Autodesk Inventor part; units mm, degrees
ref_plane "YZ Plane" through (0, 0, 0) normal (1, 0, 0) x (0, 1, 0)
ref_plane "XZ Plane" through (0, 0, 0) normal (0, 1, 0) x (-1, 0, 0)
ref_plane "XY Plane" through (0, 0, 0) normal (0, 0, 1) x (1, 0, 0)
sketch "Sketch1" plane through (0, 0, 0) normal (0, 0, 1) x (1, 0, 0)
  line L0 (-15, 70.8) -> (15, 70.8)
  line L1 (15, 70.8) -> (15, -70.8)
  line L2 (15, -70.8) -> (-15, -70.8)
  line L3 (-15, -70.8) -> (-15, 70.8)
  line L4 (0, 70.8) -> (0, -70.8) construction
  line L5 (-15, 58.8) -> (15, 58.8)
  line L6 (15, 58.8) -> (15, -58.8)
  line L7 (15, -58.8) -> (-15, -58.8)
  line L8 (-15, -58.8) -> (-15, 58.8)
  line L9 (0, 58.8) -> (0, -58.8) construction
  line L10 (-15, 58) -> (15, 58)
  line L11 (15, 58) -> (15, -58)
  line L12 (15, -58) -> (-15, -58)
  line L13 (-15, -58) -> (-15, 58)
  line L14 (0, 58) -> (0, -58) construction
  point P0 (0, 0)
  point P1 (0, 0)
  point P2 (15, -58)
  point P3 (-15, -58)
  point P4 (-15, -58.8)
  point P5 (15, -58.8)
  point P6 (-15, 58)
  point P7 (15, 58)
  point P8 (15, 58.8)
  point P9 (-15, 58.8)
  dimension "d0" = 141.6
  dimension "d1" = 30
  dimension "d4" = 117.6
  dimension "d5" = 116
extrude "Extrusion1" add sketch "Sketch1" against normal blind 0.6
extrude "Extrusion2" add sketch "Sketch1" along normal blind 5.2 contours L5 L1 L10 L3 | L12 L1 L7 L3
ref_plane "upper Plane" through (0, 0, 5.2) normal (0, 0, 1) x (1, 0, 0)
sketch "Sketch2" plane through (0, 0, 5.2) normal (0, 0, 1) x (1, 0, 0)
  line L0 (-15, 70.8) -> (15, 70.8)
  line L1 (-15, 70.8) -> (-15, 58.8)
  line L2 (-15, 58) -> (-15, -58)
  line L3 (-15, -58) -> (-15, -58.8)
  line L4 (-15, -58.8) -> (-15, -70.8)
  line L5 (-15, -70.8) -> (15, -70.8)
  line L6 (15, -70.8) -> (15, -58.8)
  line L7 (15, -58.8) -> (15, -58)
  line L8 (15, -58) -> (15, 58)
  line L9 (15, 58.8) -> (15, 70.8)
  line L10 (15, 58) -> (15, 58.8)
  line L11 (-15, 58.8) -> (-15, 58)
  line L12 (15, 58.8) -> (-15, 58.8)
  line L13 (-15, -58.8) -> (15, -58.8)
  point P0 (0, 0)
extrude "Extrusion4" add sketch "Sketch2" against normal blind 0.6 contours L0 L9 L12 L1 | L13 L6 L5 L4
equation "\"d0\" = coil_spacer_width + 2 * grab_distance"
equation "\"d1\" = coil_spacer_length"
equation "\"d4\" = coil_spacer_width"
equation "\"d5\" = coil_spacer_width - 2 * wire_diameter_tolerance"
equation "\"d2\" = coil_spacer_thickness"
equation "\"d6\" = wire_diameter"
equation "\"d11\" = coil_spacer_thickness"
equation "\"coil_spacer_length\" = 30"
equation "\"coil_spacer_width\" = 117.6"
equation "\"coil_spacer_thickness\" = 0.6"
equation "\"grab_distance\" = 12"
equation "\"wire_diameter_tolerance\" = 0.8"
equation "\"wire_diameter\" = 5.2"
properties part number "coil_spacer"
The listing builds one solid part. Answer for the finished solid, in the listing's coordinates (mm). A direction names the side the tool comes from. Coordinates: 2 decimals unless noted, no trailing zeros. Loops run counter-clockwise (first coordinate to the right, second up) from the corner with the lowest first, then second, coordinate; pieces in that order, holes last. Notation, with made-up numbers: (-4.75, 78) - (29.25, 78) arc R22 ccw to (29.25, 112) - close; hole circle Ø9 at (65, 45.5). An arc over 180 degrees is marked (long way). Use a Markdown table: item, result. Add a question column.
1) The mould has two halves that part along Y. Classify faces 1 (the flat face through (0, -58, 3)), 2 (the flat face through (0, -58.8, 2)), 3 (the flat face through (15, 16.1, -0.3)), 4 (the flat face through (0, 58, 3)): released by +Y, released by -Y, zero draft, split by the parting line, or undercut.
2) For faces 5 (the flat face through (0, 1, 0)), 6 (the flat face through (0, -65, 4.6)), 7 (the flat face through (0, 65, 0)), determine the directions among +Z, -Z, +X, -X, +Y, -Y from which every point of the face is accessible in a straight line to the end or side of a thin tool.
3) Given pin 1 (15 mm diameter, centred on x = 4.5, y = -0.5, fed in from +Z); pin 2 (1 mm diameter, centred on y = -34.5, z = 1.5, fed in from -X), each flat-ended and moving along its own axis, determine where each tip first touches the part or whether it passes through.
4) The part is cut by section B-B, the plane x = 2.5. Give the vertices of the cut face in (y, z), and give its area (3 significant figures).
5) Find the intervals of material crossed by line 1 (Z direction, x = -7, y = 59); line 2 (Y direction, x = 10.75, z = 3.8); line 3 (Z direction, x = -3, y = -13), in increasing order.
6) The part is cut by section A-A, the plane z = 1.85. Give the vertices of the cut face in (x, y).
7) The part is cut by section C-C, the plane y = 47.5. Give the vertices of the cut face in (x, z), and give its area (3 significant figures).
Here are the results:
| question | item | result |
|---|---|---|
| 1 | face 1 | undercut |
| 1 | face 2 | released by -Y |
| 1 | face 3 | zero draft |
| 1 | face 4 | undercut |
| 2 | face 5 | +Z, +X, -X |
| 2 | face 6 | +X, -X, -Y |
| 2 | face 7 | +X, -X, +Y |
| 3 | pin 1 | stops at z = 0 |
| 3 | pin 2 | passes through |
| 4 | outline | (-70.8, -0.6) - (70.8, -0.6) - (70.8, 0) - (58.8, 0) - (58.8, 4.6) - (70.8, 4.6) - (70.8, 5.2) - (58, 5.2) - (58, 0) - (-58, 0) - (-58, 5.2) - (-70.8, 5.2) - (-70.8, 4.6) - (-58.8, 4.6) - (-58.8, 0) - (-70.8, 0) - close |
| 4 | area | 108 mm^2 |
| 5 | line 1 | z = -0.6 to 0, 4.6 to 5.2 |
| 5 | line 2 | y = -58.8 to -58, 58 to 58.8 |
| 5 | line 3 | z = -0.6 to 0 |
| 6 | outline | (-15, -58.8) - (15, -58.8) - (15, -58) - (-15, -58) - close; (-15, 58) - (15, 58) - (15, 58.8) - (-15, 58.8) - close |
| 7 | outline | (-15, -0.6) - (15, -0.6) - (15, 0) - (-15, 0) - close |
| 7 | area | 18.0 mm^2 |
